The drawing under review shows one solid part. Ordinate dimensions are in mm from its lowest x, y, z. A direction names the side the tool comes from. Round coordinates to 2 decimals unless told otherwise and drop trailing zeros. Write each loop counter-clockwise with the first axis right and the second up, starting at its lowest first coordinate (ties: lowest second). Pieces come first, ordered by that corner, then holes.
Item 1: Machinability: for the marked faces 5, 6 and 7, which of the approach directions +Z, -Z, +X, -X, +Y, -Y give a long, thin tool a straight path to every point of the face, cutting with its end or side? Answer none if there is none.
Item 2: Add section D-D (y = 4). Give the boundary of the cut face in (x, z) (3 decimals), plus the area to 3 significant figures.
Item 3: Clearance check with flat-ended pins moving along their axes: pin 1 Ø6 at (y, z) = (9, 13) entering from -X; pin 2 Ø3 at (y, z) = (18.5, 2.5) entering from -X; pin 3 Ø4 at (y, z) = (21.5, 11) entering from +X (3 decimals). State where each tip first meets the part, or that it passes through.
Item 4: Add section B-B (x = 15). Give the boundary of the cut face in (y, z) (3 decimals), plus the area to 3 significant figures.
Item 5: Add section A-A (z = 6.75). Give the boundary of the cut face in (x, y) (3 decimals).
Item 6: Draft analysis for pull direction Z (two halves, no side actions). For the marked faces 1, 2, 3 and 4, state which applies: +Z half, -Z half, draft (parallel to the pull), parting line (faces both ways), or undercut.
Item 7: To check wall thickness, follow L1, parallel to Z at x = 11, y = 4.75 (3 decimals); L2, parallel to Z at x = 6.5, y = 14; L3, parallel to Y at x = 19.5, z = 1.5 (3 decimals). State the ranges of each line that lie inside material, in increasing order.
Item 8: Add section C-C (z = 16). Give the boundary of the cut face in (x, y) (3 decimals).
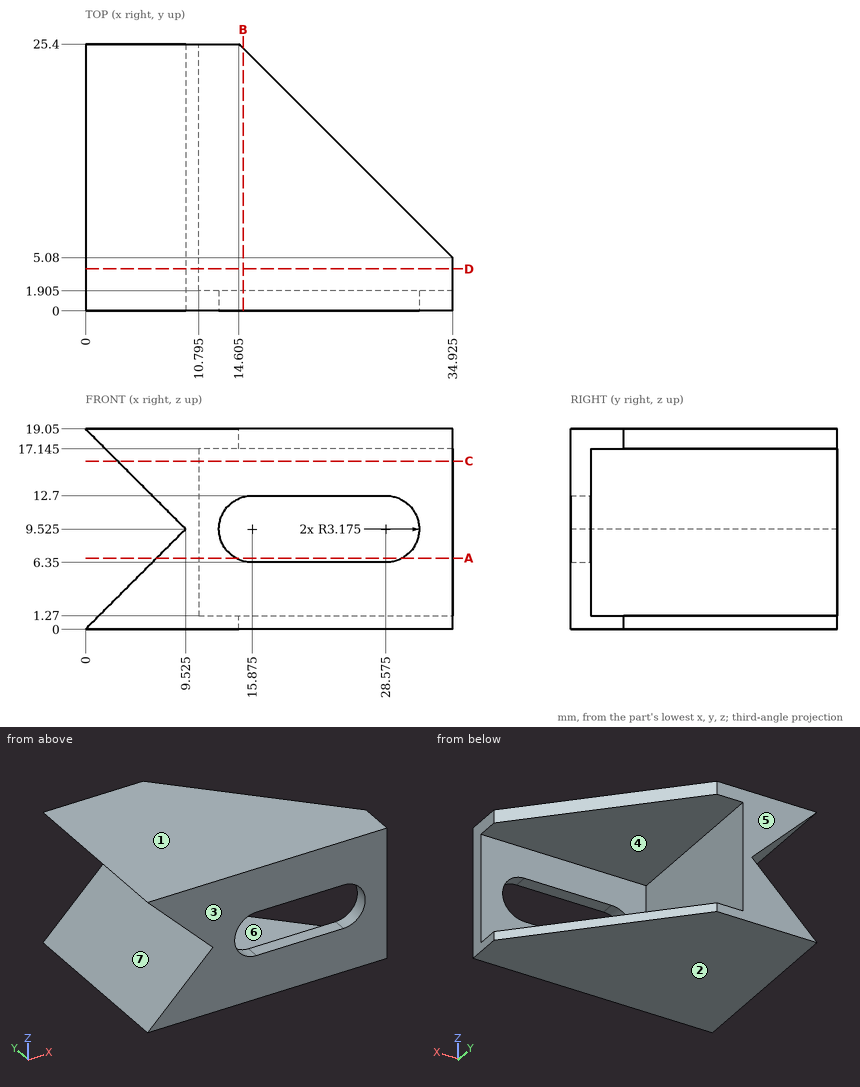
Numbers:
1. face 5: +Z, -Z, +X, -X, +Y
1. face 6: +X, +Y
1. face 7: -X, +Y, -Y
2. outline: (0, 0) - (34.925, 0) - (34.925, 1.27) - (10.795, 1.27) - (10.795, 17.145) - (34.925, 17.145) - (34.925, 19.05) - (0, 19.05) - (9.525, 9.525) - close
2. area: 192 mm2
3. pin 1: stops at x = 3.05
3. pin 2: stops at x = 1
3. pin 3: stops at x = 10.795
4. outline: (0, 0) - (25.005, 0) - (25.005, 1.27) - (1.905, 1.27) - (1.905, 6.473) - (0, 6.473) - close; (0, 12.577) - (1.905, 12.577) - (1.905, 17.145) - (25.005, 17.145) - (25.005, 19.05) - (0, 19.05) - close
4. area: 98.0 mm2
5. outline: (6.75, 0) - (14.332, 0) - (14.332, 1.905) - (10.795, 1.905) - (10.795, 25.4) - (6.75, 25.4) - close; (30.118, 0) - (34.925, 0) - (34.925, 1.905) - (30.118, 1.905) - close
6. face 1: +Z half
6. face 2: -Z half
6. face 3: draft
6. face 4: undercut
7. L1: z = 0 to 1.27, 17.145 to 19.05
7. L2: z = 0 to 6.5, 12.55 to 19.05
7. L3: y = 0 to 1.905
8. outline: (3.05, 0) - (34.925, 0) - (34.925, 1.905) - (10.795, 1.905) - (10.795, 25.4) - (3.05, 25.4) - close
